from build123d import *

# Parameters (mm, degrees)
BOSS_EXTRUDE1_DEPTH = 1.6
SKETCH2_W           = 8.35
SKETCH2_H           = 7
SKETCH2_W_2         = 10
SKETCH2_H_2         = 10
BOSS_EXTRUDE2_DEPTH = 1.9
FILLET1_R           = 0.7


with BuildPart() as part:
    # Sketch1 → Boss-Extrude1 (new body)
    with BuildSketch(Plane(origin=(0, 0, 0), x_dir=(1, 0, 0), z_dir=(0, 1, 0))):
        with BuildLine():
            Line((7.4, 0), (-7.4, 0))
            ThreePointArc((-7.4, 0), (-8.460660172, 0.439339828), (-8.9, 1.5))
            Line((-8.9, 1.5), (-8.9, 19.5))
            ThreePointArc((-8.9, 19.5), (-8.460660172, 20.560660172), (-7.4, 21))
            Line((-7.4, 21), (7.4, 21))
            ThreePointArc((7.4, 21), (8.460660172, 20.560660172), (8.9, 19.5))
            Line((8.9, 19.5), (8.9, 1.5))
            ThreePointArc((8.9, 1.5), (8.460660172, 0.439339828), (7.4, 0))
        make_face()
    extrude(amount=BOSS_EXTRUDE1_DEPTH)

    # Sketch2 → Boss-Extrude2 (add)
    with BuildSketch(Plane(origin=(0, 1.6, 0), x_dir=(1, 0, 0), z_dir=(0, 1, 0))):
        with Locations((0, 19)):
            Rectangle(SKETCH2_W, SKETCH2_H)
        with Locations((0, 8.5)):
            Rectangle(SKETCH2_W_2, SKETCH2_H_2)
    extrude(amount=BOSS_EXTRUDE2_DEPTH)

    # Fillet1
    fillet1_edges = [part.edges().sort_by_distance(p)[0] for p in [
        (-4.175, 1.6, -21.75),
        (4.175, 1.6, -21.75),
        (-4.175, 3.5, -19),
        (4.175, 3.5, -19),
    ]]
    fillet(fillet1_edges, radius=FILLET1_R)


solid = part.part
Design review of the part built by this model. Coordinates are the model's own, in mm. A direction names the side the tool comes from. Coordinates: 2 decimals unless noted, no trailing zeros. Loops run counter-clockwise (first coordinate to the right, second up) from the corner with the lowest first, then second, coordinate; pieces in that order, holes last.
Item 1: Add section C-C (x = 1.5). Write out the cut boundary in (y, z).
Completed:
outline: (0, -21) - (1.6, -21) - (1.6, -22.5) - (3.5, -22.5) - (3.5, -15.5) - (1.6, -15.5) - (1.6, -13.5) - (3.5, -13.5) - (3.5, -3.5) - (1.6, -3.5) - (1.6, 0) - (0, 0) - close
Item 2: For faces 4 (the flat face through (4.175, 2, -19)), 5 (the flat face through (5, 3, -8)), 6 (the flat face through (0, 3, -13.5)), 7 (the cylindrical face through (8.45, 0.79, -20.57)), list the 3-axis set-ups (+Z, -Z, +X, -X, +Y, -Y) from which the entire face can be reached by the end or side of a thin tool; tool diameter is ignored.
Completed:
face 4: -Z, +X, +Y
face 5: +Z, -Z, +X, +Y
face 6: +X, -X, +Y
face 7: -Z, +X, +Y, -Y
Item 3: Add section A-A (x = -4.5). Write out the cut boundary in (y, z).
Completed:
outline: (0, -21) - (1.6, -21) - (1.6, -13.5) - (3.5, -13.5) - (3.5, -3.5) - (1.6, -3.5) - (1.6, 0) - (0, 0) - close
Item 4: Clearance check with flat-ended pins moving along their axes: pin 1 (1.5 mm diameter, centred on y = 2.5, z = -17, fed in from -X) (3 decimals); pin 2 (1.5 mm diameter, centred on y = 2.5, z = -10.5, fed in from -X); pin 3 (1.3 mm diameter, centred on y = 2.5, z = -19.5, fed in from +X) (3 decimals). State where each tip first meets the part, or that it passes through.
Completed:
pin 1: stops at x = -4.175
pin 2: stops at x = -5
pin 3: stops at x = 4.175
Item 5: Add section B-B (z = -11.5). Write out the cut boundary in (x, y), and give its area (3 significant figures).
Completed:
outline: (-8.9, 0) - (8.9, 0) - (8.9, 1.6) - (5, 1.6) - (5, 3.5) - (-5, 3.5) - (-5, 1.6) - (-8.9, 1.6) - close
area: 47.5 mm2
Item 6: Draft analysis for pull direction Z (two halves, no side actions). For faces 1 (the flat face through (0, 3, -15.5)), 2 (the flat face through (-5, 3, -8)), 3 (the flat face through (0, 3, -3.5)), state which applies: pulls with the +Z half, pulls with the -Z half, needs draft (parallel to the pull), parting line crosses it, or undercut.
Completed:
face 1: undercut
face 2: needs draft
face 3: pulls with the +Z half
Item 7: Wall thickness on L1, parallel to Z at x = -1.75, y = 2.1; L2, parallel to Y at x = 7.75, z = -20; L3, parallel to X at y = 2.75, z = -7.5: over which ranges is each line inside the solid? List them lowest first.
Completed:
L1: z = -22.5 to -15.5, -13.5 to -3.5
L2: y = 0 to 1.6
L3: x = -5 to 5
Item 8: Add section D-D (z = -19.25). Write out the cut boundary in (x, y) (3 decimals), and give its area (3 significant figures).
Completed:
outline: (-8.9, 0) - (8.9, 0) - (8.9, 1.6) - (4.175, 1.6) - (4.175, 2.8) arc R0.7 ccw to (3.475, 3.5) - (-3.475, 3.5) arc R0.7 ccw to (-4.175, 2.8) - (-4.175, 1.6) - (-8.9, 1.6) - close
area: 44.1 mm2
